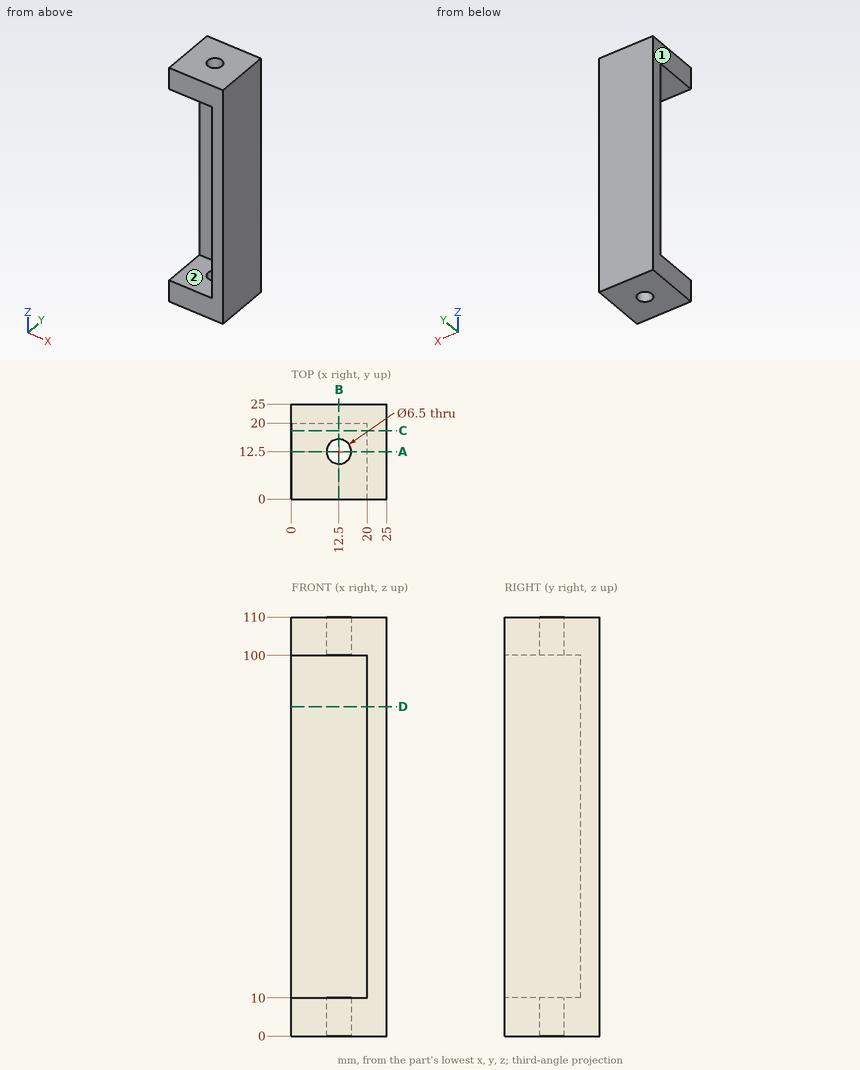
Print and shaded views of the part. All mm, measured from the part's lowest x, y and z. A direction names the side the tool comes from. Coordinates: 2 decimals unless noted, no trailing zeros. Write each loop counter-clockwise with the first axis right and the second up, starting at its lowest first coordinate (ties: lowest second). Pieces come first, ordered by that corner, then holes.
(1) Cut at A-A, the plane y = 12.5. List the corners of the cut face in (x, z), and give its area (3 significant figures).
(2) Drill centre lines: probe 1 along Z at (x, y) = (2.5, 12.5); probe 2 along Y at (x, z) = (12.5, 7); probe 3 along Y at (x, z) = (7.75, 56). Where is each one in solid material? Low to high.
(3) Flat gauge pins, fed straight in: pin 1 (6 mm diameter, centred on y = 7.5, z = 38, fed in from -X); pin 2 (5 mm diameter, centred on x = 10, z = 34, fed in from -Y); pin 3 (6 mm diameter, centred on x = 12.5, y = 12.5, fed in from -Z). Where does each tip first touch, or does it go through?
(4) Cut at C-C, the plane y = 18. List the corners of the cut face in (x, z).
(5) 3-axis set-ups, long thin cutter, end or side, ignore diameter. For the marked faces 1 and 2: which of +Z, -Z, +X, -X, +Y, -Y reach the whole face in a straight line?
(6) Cut at D-D, the plane z = 86.5. List the corners of the cut face in (x, y).
Geometry says:
1. outline: (0, 0) - (9.25, 0) - (9.25, 10) - (0, 10) - close; (0, 100) - (9.25, 100) - (9.25, 110) - (0, 110) - close; (15.75, 0) - (25, 0) - (25, 110) - (15.75, 110) - (15.75, 100) - (20, 100) - (20, 10) - (15.75, 10) - close
1. area: 820 mm2
2. probe 1: z = 0 to 10, 100 to 110
2. probe 2: y = 0 to 9.25, 15.75 to 25
2. probe 3: y = 20 to 25
3. pin 1: stops at x = 20
3. pin 2: stops at y = 20
3. pin 3: passes through
4. outline: (0, 0) - (25, 0) - (25, 110) - (0, 110) - (0, 100) - (20, 100) - (20, 10) - (0, 10) - close
5. face 1: +Z, -Z, -X, +Y, -Y
5. face 2: -X, -Y
6. outline: (0, 20) - (20, 20) - (20, 0) - (25, 0) - (25, 25) - (0, 25) - close
